Here's how the part is built. I have some questions about the finished solid (model axes, mm). A direction names the side the tool comes from. Round coordinates to 2 decimals unless told otherwise and drop trailing zeros. Loops run counter-clockwise (first coordinate to the right, second up) from the corner with the lowest first, then second, coordinate; pieces in that order, holes last. Notation, with made-up numbers: M -3,59.25 L 24,59.25 A25 cw 24,82.25 Z; hole C 72,-33.5 d7. An arc over 180 degrees is marked long. Answer as a JSON object with one key per item and string values.
Autodesk Inventor part; units mm, degrees
ref_plane "YZ Plane" through (0, 0, 0) normal (1, 0, 0) x (0, 1, 0)
ref_plane "XZ Plane" through (0, 0, 0) normal (0, 1, 0) x (-1, 0, 0)
ref_plane "XY Plane" through (0, 0, 0) normal (0, 0, 1) x (1, 0, 0)
sketch "Skizze1" plane through (0, 0, 0) normal (0, 0, 1) x (1, 0, 0)
  line L0 (-24.0065, 29.05) -> (24.0065, 29.05)
  line L1 (24.0065, 29.05) -> (24.0065, -29.05)
  line L2 (24.0065, -29.05) -> (-24.0065, -29.05)
  line L3 (-24.0065, -29.05) -> (-24.0065, 29.05)
  line L4 (-24.0065, 29.05) -> (24.0065, -29.05) construction
  line L5 (24.0065, 29.05) -> (-24.0065, -29.05) construction
  line L6 (-24.0065, 29.05) -> (-20.0065, 29.05)
  line L7 (-20.0065, 29.05) -> (-20.0065, -29.05)
  line L8 (-20.0065, -29.05) -> (-24.0065, -29.05)
  line L9 (-24.0065, -29.05) -> (-24.0065, 29.05)
  line L10 (-20.0065, -29.05) -> (24.0065, -29.05)
  line L11 (24.0065, -29.05) -> (24.0065, -25.05)
  line L12 (24.0065, -25.05) -> (-20.0065, -25.05)
  line L13 (-20.0065, -25.05) -> (-20.0065, -29.05)
  line L14 (24.0065, -25.05) -> (20.0065, -25.05)
  line L15 (20.0065, -25.05) -> (20.0065, 29.05)
  line L16 (20.0065, 29.05) -> (24.0065, 29.05)
  line L17 (24.0065, 29.05) -> (24.0065, -25.05)
  line L18 (20.0065, 29.05) -> (-20.0065, 29.05)
  line L19 (-20.0065, 29.05) -> (-20.0065, 25.05)
  line L20 (-20.0065, 25.05) -> (20.0065, 25.05)
  line L21 (20.0065, 25.05) -> (20.0065, 29.05)
  line L22 (-20.0065, 25.05) -> (20.0065, 25.05)
  line L23 (20.0065, 25.05) -> (20.0065, 23.05)
  line L24 (20.0065, 23.05) -> (-20.0065, 23.05)
  line L25 (-20.0065, 23.05) -> (-20.0065, 25.05)
  line L26 (-20.0065, -25.05) -> (20.0065, -25.05)
  line L27 (20.0065, -25.05) -> (20.0065, -23.05)
  line L28 (20.0065, -23.05) -> (-20.0065, -23.05)
  line L29 (-20.0065, -23.05) -> (-20.0065, -25.05)
  line L30 (-24.0065, 29.05) -> (24.0065, 29.05)
  line L31 (24.0065, 29.05) -> (24.0065, -29.05)
  line L32 (24.0065, -29.05) -> (-24.0065, -29.05)
  line L33 (-24.0065, -29.05) -> (-24.0065, 29.05)
  circle A0 centre (-14.7085, 19.65) radius 1.35
  circle A1 centre (15.6927, 19.65) radius 1.35
  circle A2 centre (-14.7085, -8.9604) radius 1.35
  circle A3 centre (15.6927, -8.9604) radius 1.35
  line L34 (-17.3399, 17.2285) -> (18.4839, 17.2285)
  line L35 (18.4839, 17.2285) -> (18.4839, -6.4884)
  line L36 (18.4839, -6.4884) -> (-17.3399, -6.4884)
  line L37 (-17.3399, -6.4884) -> (-17.3399, 17.2285)
  line L38 (-17.3399, -6.4884) -> (-6.9094, -6.4884)
  line L39 (-6.9094, -10.3104) -> (-6.9094, -6.4884)
  line L40 (18.4839, -6.4884) -> (8.0539, -6.4884)
  line L41 (8.0539, -6.4884) -> (8.0539, -10.3104)
  line L42 (8.0539, -10.3104) -> (-6.9094, -10.3104)
  line L43 (-6.9094, 22.1958) -> (8.0539, 22.1958)
  line L44 (8.0539, 22.1958) -> (8.0539, 17.8498)
  line L45 (8.0539, 17.8498) -> (-6.9094, 17.8498)
  line L46 (-6.9094, 17.8498) -> (-6.9094, 22.1958)
  point P0 (0, 0)
  point P1 (-20.0065, -25.05)
  dimension "d0" = 48.013
  dimension "d1" = 58.1
  dimension "d2" = 4
  dimension "d3" = 4
  dimension "d4" = 4
  dimension "d5" = 4
  dimension "d6" = 2
  dimension "d7" = 2
  dimension "d28" = 2.7
  dimension "d29" = 2.7
  dimension "d30" = 2.7
  dimension "d31" = 2.7
  dimension "d32" = 10.43
  dimension "d33" = 3.822
extrude "Extrusion1" add sketch "Skizze1" against normal blind 7 contours L20 L15 L24 L7 | L7 L28 L15 L12
sketch "Skizze2" plane through (-20.0065, -25.05, 0) normal (0, -1, 0) x (1, 0, 0)
  line L0 (40.013, 0) -> (0, 0)
  line L1 (40.013, 0) -> (20.013, 0)
  line L2 (20.013, 0) -> (20.013, -5)
  line L3 (15.513, -3.2) -> (24.513, -3.2)
  line L4 (24.513, -3.2) -> (24.513, -6.8)
  line L5 (24.513, -6.8) -> (15.513, -6.8)
  line L6 (15.513, -6.8) -> (15.513, -3.2)
  line L7 (15.513, -3.2) -> (24.513, -6.8) construction
  line L8 (24.513, -3.2) -> (15.513, -6.8) construction
  line L9 (20.013, -5) -> (15.513, -5)
  line L10 (20.013, -5) -> (24.513, -5)
  point P0 (20.0065, 0)
  dimension "d10" = 20
  dimension "d11" = 5
  dimension "d12" = 9
  dimension "d13" = 3.6
extrude "Extrusion2" add sketch "Skizze2" along normal blind 1.8
chamfer "Fasen1" distance 1.8 angle 45 2 edges at (0.0065, -26.85, -3.2) (0.0065, -26.85, -6.8)
sketch "Skizze3" plane through (-20.0065, 25.05, 0) normal (0, 1, 0) x (1, 0, 0)
  line L0 (40.013, 0) -> (40.013, 7)
  line L1 (40.013, 0) -> (20.013, 0)
  line L2 (0, 0) -> (40.013, 0)
  line L3 (20.013, 0) -> (20.013, 5)
  line L4 (24.513, 3.2) -> (15.513, 3.2)
  line L5 (15.513, 3.2) -> (15.513, 6.8)
  line L6 (15.513, 6.8) -> (24.513, 6.8)
  line L7 (24.513, 6.8) -> (24.513, 3.2)
  line L8 (24.513, 3.2) -> (15.513, 6.8) construction
  line L9 (15.513, 3.2) -> (24.513, 6.8) construction
  line L10 (20.013, 5) -> (24.513, 5)
  line L11 (24.513, 5) -> (15.513, 5)
  line L12 (15.513, 5) -> (15.513, 6.8)
  line L13 (15.513, 6.8) -> (24.513, 6.8)
  line L14 (24.513, 6.8) -> (24.513, 5)
  point P0 (20.0065, 0)
  dimension "d19" = 20
  dimension "d20" = 5
  dimension "d21" = 9
  dimension "d22" = 3.6
extrude "Extrusion3" add sketch "Skizze3" along normal blind 1.8
chamfer "Fasen2" distance 1.8 angle 45 2 edges at (0.0065, 26.85, -3.2) (0.0065, 26.85, -6.8)
extrude "Extrusion4" add sketch "Skizze1" along normal blind 4 contours L0 L7 L2 L3 | L0 L15 L20 L7 | L0 L1 L12 L15 | L20 L15 L24 L7 | L7 L12 L1 L2 | L24 L15 L28 L7 | L7 L28 L15 L12 | A0 | A1 | A2 | A3 | L34 L35 L36 L37 | L36 L41 L42 L39 | L43 L44 L45 L46
extrude "Extrusion5" add sketch "Skizze1" against normal blind 3 contours A0 | A1 | A2 | A3
extrude "Extrusion6" cut sketch "Skizze1" along normal blind 4 contours L34 L35 L36 L37 | L36 L41 L42 L39
fillet "Rundung1" radius 1 16 edges at (0.572, 17.2285, 4) (-17.3399, 5.3701, 4) (-12.1246, -6.4884, 4) (-6.9094, -8.3994, 4) (0.5723, -10.3104, 4) (8.0539, -8.3994, 4) (13.2689, -6.4884, 4) (18.4839, 5.3701, 4) (8.0539, -8.3994, 0) (13.2689, -6.4884, 0) (18.4839, 5.3701, 0) (0.5723, -10.3104, 0) (-12.1246, -6.4884, 0) (-6.9094, -8.3994, 0) (-17.3399, 5.3701, 0) (0.572, 17.2285, 0)
extrude "Extrusion7" cut sketch "Skizze1" along normal blind 3 contours L43 L44 L45 L46
sketch "Skizze4" plane through (0, 0, 0) normal (0, 0, -1) x (-1, 0, 0)
  line L0 (-17.7346, -15.3743) -> (-10.7346, -15.3743)
  line L1 (-10.7346, -15.3743) -> (-10.7346, -22.3743)
  line L2 (-10.7346, -22.3743) -> (-17.7346, -22.3743)
  line L3 (-17.7346, -22.3743) -> (-17.7346, -15.3743)
  line L4 (-17.7346, -15.3743) -> (-10.7346, -22.3743) construction
  line L5 (-10.7346, -15.3743) -> (-17.7346, -22.3743) construction
  line L6 (-18.7346, -14.3743) -> (-9.7346, -14.3743)
  line L7 (-9.7346, -14.3743) -> (-9.7346, -23.3743)
  line L8 (-9.7346, -23.3743) -> (-18.7346, -23.3743)
  line L9 (-18.7346, -23.3743) -> (-18.7346, -14.3743)
  line L10 (-18.7346, -14.3743) -> (-9.7346, -23.3743) construction
  line L11 (-9.7346, -14.3743) -> (-18.7346, -23.3743) construction
  line L12 (-17.2346, -15.8743) -> (-11.2346, -15.8743)
  line L13 (-11.2346, -15.8743) -> (-11.2346, -21.8743)
  line L14 (-11.2346, -21.8743) -> (-17.2346, -21.8743)
  line L15 (-17.2346, -21.8743) -> (-17.2346, -15.8743)
  line L16 (-17.2346, -15.8743) -> (-11.2346, -21.8743) construction
  line L17 (-11.2346, -15.8743) -> (-17.2346, -21.8743) construction
  line L18 (9.178, -15.8743) -> (15.178, -15.8743)
  line L19 (15.178, -15.8743) -> (15.178, -21.8743)
  line L20 (15.178, -21.8743) -> (9.178, -21.8743)
  line L21 (9.178, -21.8743) -> (9.178, -15.8743)
  line L22 (9.178, -15.8743) -> (15.178, -21.8743) construction
  line L23 (15.178, -15.8743) -> (9.178, -21.8743) construction
  line L24 (8.678, -15.3743) -> (15.678, -15.3743)
  line L25 (15.678, -15.3743) -> (15.678, -22.3743)
  line L26 (15.678, -22.3743) -> (8.678, -22.3743)
  line L27 (8.678, -22.3743) -> (8.678, -15.3743)
  line L28 (8.678, -15.3743) -> (15.678, -22.3743) construction
  line L29 (15.678, -15.3743) -> (8.678, -22.3743) construction
  line L30 (7.678, -14.3743) -> (16.678, -14.3743)
  line L31 (16.678, -14.3743) -> (16.678, -23.3743)
  line L32 (16.678, -23.3743) -> (7.678, -23.3743)
  line L33 (7.678, -23.3743) -> (7.678, -14.3743)
  line L34 (7.678, -14.3743) -> (16.678, -23.3743) construction
  line L35 (16.678, -14.3743) -> (7.678, -23.3743) construction
  point P0 (0, 0)
  point P1 (-14.2346, -18.8743)
  point P2 (-14.2346, -18.8743)
  point P3 (-14.2346, -18.8743)
  point P4 (12.178, -18.8743)
  point P5 (12.178, -18.8743)
  point P6 (12.178, -18.8743)
  dimension "d43" = 7
  dimension "d44" = 7
  dimension "d45" = 9
  dimension "d46" = 9
  dimension "d47" = 6
  dimension "d48" = 6
  dimension "d49" = 6
  dimension "d50" = 6
  dimension "d51" = 7
  dimension "d52" = 7
  dimension "d53" = 9
  dimension "d54" = 9
extrude "Extrusion8" add sketch "Skizze4" along normal blind 5 contours L6 L7 L8 L9 | L30 L31 L32 L33
extrude "Extrusion9" add sketch "Skizze4" along normal blind 2 contours L0 L1 L2 L3 | L24 L25 L26 L27
extrude "Extrusion10" cut sketch "Skizze4" against normal blind 5 contours L12 L13 L14 L15 | L18 L19 L20 L21
fillet "Rundung2" radius 1 12 edges at (-12.178, -15.8743, 4) (-9.178, -18.8743, 4) (-12.178, -21.8743, 4) (-15.178, -18.8743, 4) (11.2346, -18.8743, 4) (14.2346, -15.8743, 4) (17.2346, -18.8743, 4) (14.2346, -21.8743, 4) (-24.0065, 0, 4) (0, -29.05, 4) (24.0065, 0, 4) (0, 29.05, 4)
properties part number "Deckel"
Item 1: We'd pull the mould along X, two halves only. Please class faces 1 (the face through (16, 20, -3)), 2 (the face through (9.735, -19, -2)): +X half, -X half, draft (parallel to the pull), parting line (faces both ways), or undercut.
Solution:
{"face 1": "draft", "face 2": "undercut"}
Item 2: If I drill on L1, parallel to Y at x = 15, z = -4.75; L2, parallel to Y at x = 17, z = 1.5; L3, parallel to X at y = -22.5, z = -4, over which ranges is the centre line in solid material (lowest first)? Write a range as from..to.
Solution:
{"L1": "y = -25.05..-22.37, -15.37..-14.37, 23.05..25.05", "L2": "y = -29.05..-21.87, -15.87..-6.49, 17.23..29.05", "L3": "x = -16.68..-7.68, 9.73..18.73"}
Item 3: I want a section at B-B on x = -11. Count the separate pieces of the cut face and the enclosed holes in it, plus the area to 3 significant figures.
Solution:
{"separate pieces": "3", "enclosed holes": "0", "area": "150 mm2"}
Item 4: I want a section at C-C on x = 5.5. List the corners of the cut face in (y, z) for me, plus the area to 3 significant figures.
Solution:
{"outline": "M -29.05,0 L -25.05,0 L -25.05,-7 L -23.05,-7 L -23.05,0 L -11.31,0 A1 ccw -10.31,1 L -10.31,3 A1 ccw -11.31,4 L -28.05,4 A1 ccw -29.05,3 Z; M 17.23,1 A1 ccw 17.85,0.07 L 17.85,3 L 22.2,3 L 22.2,0 L 23.05,0 L 23.05,-7 L 25.05,-7 L 25.05,0 L 29.05,0 L 29.05,3 A1 ccw 28.05,4 L 18.23,4 A1 ccw 17.23,3 Z", "area": "136 mm2"}
Item 5: I want a section at D-D on z = -6. List the corners of the cut face in (x, y) for me.
Solution:
{"outline": "M -20.01,-25.05 L -4.49,-25.05 L -4.49,-25.85 L 4.51,-25.85 L 4.51,-25.05 L 20.01,-25.05 L 20.01,-23.05 L -20.01,-23.05 Z; M -20.01,23.05 L 20.01,23.05 L 20.01,25.05 L 4.51,25.05 L 4.51,25.85 L -4.49,25.85 L -4.49,25.05 L -20.01,25.05 Z"}
Item 6: For faces 3 (the face through (11, -19, -2)), 4 (the face through (14, -21.874, 0)), 5 (the face through (0.07, 25.96, -5.89)), 6 (the face through (-12, -15, -5)), 7 (the face through (0, -29.05, 1)), which set-ups out of +Z, -Z, +X, -X, +Y, -Y let a thin tool reach every point of the face, with its end or its side?
Solution:
{"face 3": "-Z", "face 4": "+Z, -Z", "face 5": "-Z, +X, -X, +Y", "face 6": "-Z, +X, -X", "face 7": "+Z, -Z, +X, -X, -Y"}
Item 7: I want a section at A-A on y = -2.5. List the corners of the cut face in (x, z) for me.
Solution:
{"outline": "M -24.01,0 L -18.34,0 A1 ccw -17.34,1 L -17.34,3 A1 ccw -18.34,4 L -23.01,4 A1 ccw -24.01,3 Z; M 18.48,1 A1 ccw 19.48,0 L 24.01,0 L 24.01,3 A1 ccw 23.01,4 L 19.48,4 A1 ccw 18.48,3 Z"}
Item 8: For P1, Ø2, axis at x = 16, y = -9.5, coming from the -Z side; P2, Ø0.5, axis at y = -26.5, z = -5.5, coming from the -X side; P3, Ø4, axis at y = -17.5, z = -2.5, coming from the -X side, each with a flat end and sliding along its axis, tell me the tip position at first contact or that it passes through.
Solution:
{"P1": "stops at z = -3", "P2": "stops at x = -4.49", "P3": "stops at x = -16.68"}
